```python
from build123d import *

# Parameters (mm, degrees)
F0_W           = 63.5
F0_H           = 38.1
F1_DEPTH       = 25.4
F2_T           = -2.54
F4_D           = 12.7
F4_CSINK_D     = 15.24
F4_CSINK_ANGLE = 90


with BuildPart() as f1:
    # F0 (on Front) → F1 (new body)
    with BuildSketch(Plane.XZ):
        with Locations((31.75, 19.05)):
            Rectangle(F0_W, F0_H)
    extrude(amount=F1_DEPTH)

    # F2
    f2_openings = [f1.faces().sort_by_distance(p)[0] for p in [
        (31.75, -25.4, 19.05),
        (31.75, -12.7, 38.1),
    ]]
    offset(amount=F2_T, openings=f2_openings)

    # F4 (through all)
    with Locations(Plane(origin=(0, 0, 0), x_dir=(-1, 0, 0), z_dir=(0, 1, 0))):
        with Locations((-31.75, 12.7)):
            CounterSinkHole(F4_D / 2, F4_CSINK_D / 2, counter_sink_angle=F4_CSINK_ANGLE)


solid = f1.part
```
For this review, take the finished solid that the model builds, in its own axes (mm). A direction names the side the tool comes from. Coordinates: 2 decimals unless noted, no trailing zeros. Loops run counter-clockwise (first coordinate to the right, second up) from the corner with the lowest first, then second, coordinate; pieces in that order, holes last.
1. Add section D-D, the plane z = 26. Give the boundary of the cut face in (x, y).
2. For faces 4 (the flat face through (63.5, -13, 19)), 5 (the flat face through (31, -14, 2.54)), list the 3-axis set-ups (+Z, -Z, +X, -X, +Y, -Y) from which the entire face can be reached by the end or side of a thin tool; tool diameter is ignored.
3. Add section B-B, the plane z = 12.7. Give the boundary of the cut face in (x, y).
4. Insertion check: P1, Ø5, axis at x = 44.5, z = 9, coming from the -Y side; P2, Ø2, axis at x = 28.5, z = 16, coming from the +Y side; P3, Ø1, axis at x = 8, y = -17, coming from the +Z side. Each pin has a flat end and moves straight along its axis. Give the tip position at first contact, or say it passes through.
5. Mouldability with a two-part tool opening along X and no side actions: class faces 1 (the flat face through (32, -25.4, 2)), 2 (the flat face through (31, -2.54, 21)), 3 (the flat face through (0, -13, 19)) as +X half, -X half, draft (parallel to the pull), parting line (faces both ways), or undercut.
6. For line 1 (Z direction, x = 31.75, y = -1.9); line 2 (X direction, y = -1.85, z = 12.7); line 3 (X direction, y = -22, z = 6), list the stretches that pass through material, from the lowest coordinate up.
7. Add section A-A, the plane x = 31.75. Give the boundary of the cut face in (y, z), then the cut area to 3 significant figures.
8. Add section C-C, the plane y = -17.5. Give the boundary of the cut face in (x, z).
Result:
1. outline: (0, -25.4) - (2.54, -25.4) - (2.54, -2.54) - (60.96, -2.54) - (60.96, -25.4) - (63.5, -25.4) - (63.5, 0) - (0, 0) - close
2. face 4: +Z, -Z, +X, +Y, -Y
2. face 5: +Z, -Y
3. outline: (0, -25.4) - (2.54, -25.4) - (2.54, -2.54) - (25.4, -2.54) - (25.4, -1.27) - (24.13, 0) - (0, 0) - close; (38.1, -2.54) - (60.96, -2.54) - (60.96, -25.4) - (63.5, -25.4) - (63.5, 0) - (39.37, 0) - (38.1, -1.27) - close
4. P1: stops at y = -2.54
4. P2: passes through
4. P3: stops at z = 2.54
5. face 1: draft
5. face 2: undercut
5. face 3: -X half
6. line 1: z = 0 to 6.35, 19.05 to 38.1
6. line 2: x = 0 to 25.4, 38.1 to 63.5
6. line 3: x = 0 to 2.54, 60.96 to 63.5
7. outline: (-25.4, 0) - (0, 0) - (0, 5.08) - (-1.27, 6.35) - (-2.54, 6.35) - (-2.54, 2.54) - (-25.4, 2.54) - close; (-2.54, 19.05) - (-1.27, 19.05) - (0, 20.32) - (0, 38.1) - (-2.54, 38.1) - close
7. area: 121 mm2
8. outline: (0, 0) - (63.5, 0) - (63.5, 38.1) - (60.96, 38.1) - (60.96, 2.54) - (2.54, 2.54) - (2.54, 38.1) - (0, 38.1) - close
